from build123d import *

# Parameters (mm, degrees)
F0_W      = 50
F0_H      = 90
F1_DEPTH  = 8
F3_DEPTH  = 49
F4_R      = 3.75
F5_DEPTH  = 25
F7_DEPTH  = 50
F9_START  = -25
F8_W      = 20
F8_H      = 14
F9_DEPTH  = 3
F11_START = 25
F11_DEPTH = 3
F13_START = 25
F12_R     = 1.0510148408
F13_DEPTH = 4
F14_SIZE  = 1.99999


# Not quite as in the source:
# - a fillet or chamfer is up to 0.001 mm smaller than in the source, because OpenCascade refuses the exact size


with BuildPart() as f1:
    # F0 (on Top) → F1 (new body)
    with BuildSketch(Plane.XY):
        Rectangle(F0_W, F0_H)
    extrude(amount=-F1_DEPTH)

    # F2 (on Top) → F3 (join)
    with BuildSketch(Plane.XY):
        Polygon((-17, 45), (-25, 45), (-25, 37), (-25, -45), (-17, -45), (-17, -40), (-21, -40), (-21, -32), (-17, -32), (-17, 37), (17, 37), (17, -32), (21, -32), (21, -40), (17, -40), (17, -45), (25, -45), (25, 37), (25, 45), (17, 45), align=None)
    extrude(amount=F3_DEPTH)

    # F4 (on Right) → F5 (cut, symmetric)
    with BuildSketch(Plane.YZ):
        with Locations((0, 42)):
            Circle(F4_R)
    extrude(amount=F5_DEPTH, both=True, mode=Mode.SUBTRACT)

    # F6 (on Front) → F7 (cut)
    with BuildSketch(Plane.XZ):
        with BuildLine():
            ThreePointArc((-12, 49), (0, 37), (12, 49))
            Line((12, 49), (-12, 49))
        make_face()
    extrude(amount=-F7_DEPTH, mode=Mode.SUBTRACT)

    # F8 (on Right) → F9 (join)
    with BuildSketch(Plane.YZ.offset(F9_START)):
        with Locations((0, 42)):
            Rectangle(F8_W, F8_H)
    extrude(amount=-F9_DEPTH)

    # F10 (on Right) → F11 (join)
    with BuildSketch(Plane.YZ.offset(F11_START)):
        with BuildLine():
            ThreePointArc((14, 42), (12.5355339059, 45.5355339059), (9, 47))
            Line((9, 47), (-14, 47))
            Line((-14, 47), (-14, 37))
            Line((-14, 37), (-12.275, 37))
            add(Edge.make_bspline(
                [(-8.722, 37), (-7.7358158763, 42.9104981706), (-9.5123158763, 42.9104981706), (-11.2888158763, 42.9104981706), (-12.275, 37)],
                knots=[4.765680137, 4.765680137, 4.765680137, 6.3364764638, 6.3364764638, 7.9072727906, 7.9072727906, 7.9072727906], degree=2, weights=[1, 0.7071067812, 1, 0.7071067812, 1]))
            Line((-8.722, 37), (9, 37))
            ThreePointArc((9, 37), (12.5355339059, 38.4644660941), (14, 42))
        make_face()
    extrude(amount=F11_DEPTH)

    # F12 (on Right) → F13 (join)
    with BuildSketch(Plane.YZ.offset(F13_START)):
        with Locations((-9.8914606497, 40.4975526035)):
            Circle(F12_R)
    extrude(amount=F13_DEPTH)

    # F14 (size 2 in the source; OpenCascade refuses exactly that, so slightly less here)
    f14_edges = [f1.edges().sort_by_distance(p)[0] for p in [
        (25, 0, -8),
        (25, -45, 20.5),
        (0, -45, -8),
        (-25, -45, 20.5),
        (-25, 0, -8),
        (-25, 45, 20.5),
        (25, 45, 20.5),
        (0, 45, -8),
        (-28, 0, 49),
        (-18.5, 45, 49),
        (18.5, 45, 49),
        (25, 0, 49),
        (-25, 27.5, 49),
        (-25, -27.5, 49),
        (-28, 10, 42),
        (-28, 0, 35),
        (-28, -10, 42),
    ]]
    chamfer(f14_edges, length=F14_SIZE)


solid = f1.part
Can you work these out from the model? Positions are in its coordinate system, mm. A direction names the side the tool comes from. Coordinates: 2 decimals unless noted, no trailing zeros. Write each loop counter-clockwise with the first axis right and the second up, starting at its lowest first coordinate (ties: lowest second). Pieces come first, ordered by that corner, then holes. Notation, with made-up numbers: (-1, 2.5) -> (51, 2.5) arc R25 cw to (51, 37.5) -> close; hole circle Ø7 at (-31.75, -33.5). An arc over 180 degrees is marked (long way). Write each question's results on one line, items separated by ' | '. Start each with the question number.
Q1. We'd pull the mould along Y, two halves only. Please class faces 6 (the face through (-23.6, 43.6, 47.8)), 7 (the face through (23.6, -43.8, -6.6)), 8 (the face through (-25, 0, 42)), 9 (the face through (-25, 1, 20)): +Y half, -Y half, draft (parallel to the pull), parting line (faces both ways), or undercut.
Q2. Imagine slicing it at B-B (z = 28). Write out the boundary of the cut face in (x, y).
Q3. I'm going to push flat-ended pins straight in: pin 1 (2.5 mm diameter, centred on x = 27, z = 42.5, fed in from -Y); pin 2 (2 mm diameter, centred on y = 30.5, z = 29.5, fed in from -X); pin 3 (5.5 mm diameter, centred on y = -42, z = 33, fed in from +X); pin 4 (21 mm diameter, centred on x = 8.5, y = -2.5, fed in from +Z). Where does each tip first touch, or does it pass through?
Q4. On a 3-axis mill with a long thin cutter (end or side, diameter ignored), from which of +Z, -Z, +X, -X, +Y, -Y can I reach the whole of each face in a straight line? I mean faces 1 (the face through (-17, 2, 24)), 2 (the face through (26, -2, 47)), 3 (the face through (-20.944, 1.73, 38.673)), 4 (the face through (-19, -45, 17)), 5 (the face through (-23.8, -43.6, -6.6)). Say none if no direction works.
Q5. Imagine slicing it at C-C (x = 0). Write out the boundary of the cut face in (y, z), then the cut area to 3 significant figures.
Q6. Imagine slicing it at A-A (x = -19). Write out the boundary of the cut face in (y, z).
Q7. If I drill on probe 1 along X at (y, z) = (4, 29.5); probe 2 along X at (y, z) = (10.5, 44.5); probe 3 along Z at (x, y) = (21.5, 0), over which ranges is the centre line in solid material (lowest first)?
Taken from the geometry:
1) face 6: +Y half | face 7: -Y half | face 8: undercut | face 9: draft
2) outline: (-25, -43) -> (-23, -45) -> (-17, -45) -> (-17, -40) -> (-21, -40) -> (-21, -32) -> (-17, -32) -> (-17, 37) -> (17, 37) -> (17, -32) -> (21, -32) -> (21, -40) -> (17, -40) -> (17, -45) -> (23, -45) -> (25, -43) -> (25, 43) -> (23, 45) -> (-23, 45) -> (-25, 43) -> close
3) pin 1: stops at y = -14 | pin 2: stops at x = -25 | pin 3: stops at x = 25 | pin 4: stops at z = 49
4) face 1: +Z, -Y | face 2: +Z, +X, +Y, -Y | face 3: none | face 4: +Z, -Z, +X, -X, -Y | face 5: -Z, -X, -Y
5) outline: (-45, -6) -> (-43, -8) -> (43, -8) -> (45, -6) -> (45, 37) -> (37, 37) -> (37, 0) -> (-45, 0) -> close | area: 1,010 mm^2
6) outline: (-45, -6) -> (-43, -8) -> (43, -8) -> (45, -6) -> (45, 47) -> (43, 49) -> (-32, 49) -> (-32, 0) -> (-40, 0) -> (-40, 49) -> (-45, 49) -> close; hole circle Ø7.5 at (0, 42)
7) probe 1: x = -25 to -17, 17 to 25 | probe 2: x = -25 to -17, 17 to 28 | probe 3: z = -8 to 38.25, 45.75 to 49
